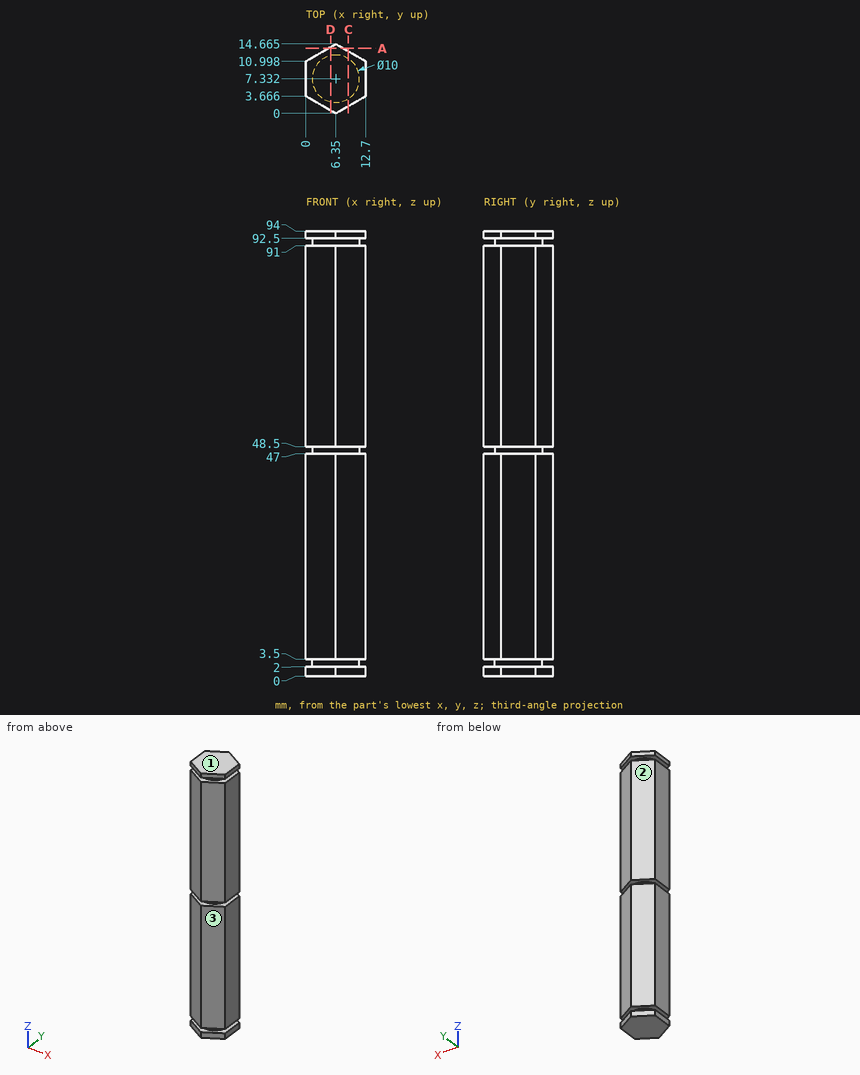
Verification items for this drawing (mm, ordinates from the low corner). Coordinates: 2 decimals unless noted, no trailing zeros. Order: outer loops, then holes, each group sorted by start corner. A loop starts at its lowest first (then second) coordinate and runs counter-clockwise, first axis right, second up. Notation, with made-up numbers: (64, 3) - (84, 3) arc R19 cw to (84, 39) - close; hole circle Ø4 at (35.5, 49). An arc over 180 degrees is marked (long way). Use one line per item in the form item = value.
1. Gauge pin test, flat ends, axial feed: pin 1 (1 mm diameter, centred on x = 5.5, z = 28.5, fed in from -Y); pin 2 (3 mm diameter, centred on x = 10, z = 34.5, fed in from +Y). Record the tip position at first contact, or that the pin passes through.
Here are the results:
pin_1 = 0.2
pin_2 = 13.42
2. Draft check along X on the marked faces 1, 2 and 3. Enter one of: pulls with the +X half, pulls with the -X half, needs draft (parallel to the pull), parting line crosses it, or undercut.
Here are the results:
face_1 = needs draft
face_2 = pulls with the -X half
face_3 = pulls with the +X half
3. Section check D-D (x = 5.25). Record the boundary of the cut face in (y, z) (1 decimal), then the cut area to 3 significant figures.
Here are the results:
outline = (0.6, 0) - (14, 0) - (14, 2) - (12.2, 2) - (12.2, 3.5) - (14, 3.5) - (14, 47) - (12.2, 47) - (12.2, 48.5) - (14, 48.5) - (14, 91) - (12.2, 91) - (12.2, 92.5) - (14, 92.5) - (14, 94) - (0.6, 94) - (0.6, 92.5) - (2.5, 92.5) - (2.5, 91) - (0.6, 91) - (0.6, 48.5) - (2.5, 48.5) - (2.5, 47) - (0.6, 47) - (0.6, 3.5) - (2.5, 3.5) - (2.5, 2) - (0.6, 2) - close
area = 1,240 mm²
4. Section check A-A (y = 13.75). Record the boundary of the cut face in (x, z) (1 decimal).
Here are the results:
outline = (4.8, 0) - (7.9, 0) - (7.9, 2) - (4.8, 2) - close; (4.8, 3.5) - (7.9, 3.5) - (7.9, 47) - (4.8, 47) - close; (4.8, 48.5) - (7.9, 48.5) - (7.9, 91) - (4.8, 91) - close; (4.8, 92.5) - (7.9, 92.5) - (7.9, 94) - (4.8, 94) - close
5. Section check C-C (x = 9). Record the boundary of the cut face in (y, z) (1 decimal).
Here are the results:
outline = (1.5, 0) - (13.1, 0) - (13.1, 2) - (11.6, 2) - (11.6, 3.5) - (13.1, 3.5) - (13.1, 47) - (11.6, 47) - (11.6, 48.5) - (13.1, 48.5) - (13.1, 91) - (11.6, 91) - (11.6, 92.5) - (13.1, 92.5) - (13.1, 94) - (1.5, 94) - (1.5, 92.5) - (3.1, 92.5) - (3.1, 91) - (1.5, 91) - (1.5, 48.5) - (3.1, 48.5) - (3.1, 47) - (1.5, 47) - (1.5, 3.5) - (3.1, 3.5) - (3.1, 2) - (1.5, 2) - close
6. Scan lines: line 1 (Z direction, x = 6.75, y = 2.25); line 2 (X direction, y = 11, z = 29) (1 decimal); line 3 (Y direction, x = 2, z = 54.5) (1 decimal). Record each from-to range of solid material in increasing order.
Here are the results:
line_1 = 0 to 2, 3.5 to 47, 48.5 to 91, 92.5 to 94
line_2 = 0 to 12.7
line_3 = 2.5 to 12.2
